Input: part model. Units: mm. Frame: model coordinates. Give positions to 0.01 mm unless a question says otherwise; leave off trailing zeros. Write each loop counter-clockwise with the first axis right and the second up, starting at its lowest first coordinate (ties: lowest second). Pieces come first, ordered by that corner, then holes. Notation, with made-up numbers: (59.25, 14.25) - (79.25, 14.25) arc R16 ccw to (79.25, 41.25) - close; hole circle Ø7 at (36, 88). An arc over 180 degrees is marked (long way). Answer as a JSON object with one key per item and string values. Group by question number.
from build123d import *

# Parameters (mm, degrees)
SKETCH2_R           = 1.5
SKETCH2_W           = 40
SKETCH2_H           = 20
SKETCH2_W_2         = 10
SKETCH2_H_2         = 3
BOSS_EXTRUDE1_DEPTH = 3


with BuildPart() as part:
    # Sketch2 → Boss-Extrude1 (new body)
    with BuildSketch(Plane(origin=(0, 0, 0), x_dir=(1, 0, 0), z_dir=(0, 1, 0))):
        Polygon((0, 15.5), (5, 15.5), (5, 47.5), (-45, 47.5), (-45, 15.5), (-40, 15.5), (-40, 0), (-36, 0), (-36, -3), (-26, -3), (-26, 0), (-21.5, 0), (-21.5, 3.1), (-22.8, 3.1), (-22.8, 5.6), (-21.5, 5.6), (-21.5, 9.4), (-18.5, 9.4), (-18.5, 5.6), (-17.2, 5.6), (-17.2, 3.1), (-18.5, 3.1), (-18.5, 0), (-14, 0), (-14, -3), (-4, -3), (-4, 0), (0, 0), align=None)
        with Locations(Location((-7.5, 15.5, 0), (0, 0, 270))):
            Circle(SKETCH2_R, mode=Mode.SUBTRACT)
        with Locations(Location((-32.5, 15.5, 0), (0, 0, 270))):
            Circle(SKETCH2_R, mode=Mode.SUBTRACT)
        with Locations(Location((-30.75, 7.9, 0), (0, 0, 270))):
            Circle(SKETCH2_R, mode=Mode.SUBTRACT)
        with Locations((-20, 31.5)):
            Rectangle(SKETCH2_W, SKETCH2_H, mode=Mode.SUBTRACT)
        with Locations((-20, 15.5)):
            Rectangle(SKETCH2_W_2, SKETCH2_H_2, mode=Mode.SUBTRACT)
        with Locations((-9, 7.9)):
            Rectangle(SKETCH2_W_2, SKETCH2_H_2, mode=Mode.SUBTRACT)
    extrude(amount=BOSS_EXTRUDE1_DEPTH)


solid = part.part
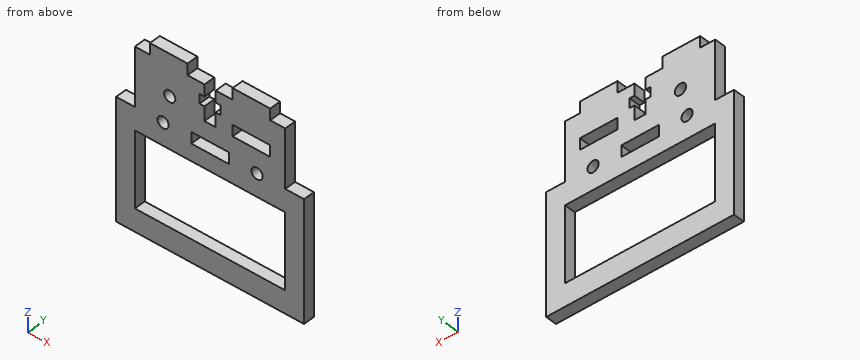
1) Cut plane D-D on y = 2.35. Count the separate pieces of the cut face and the enclosed holes in it, and give its area (3 significant figures).
2) Cut plane B-B on x = -7.5. Return the cut outline in (y, z), and give its area (3 significant figures).
3) Pin query (flat end, axial travel): P1, Ø1.5, axis at x = -24.5, y = 2, coming from the +Z side; P2, Ø0.7, axis at y = 2, z = -4, coming from the +X side; P3, Ø1.8, axis at x = -30.75, z = -7.9, coming from the +Y side. Return the tip coordinate at first contact, or that it passes through.
4) Cut plane A-A on z = -7.9. Return the cut outline in (x, y).
5) Line query: line 1 along X through (y, z) = (1.6, -7.9); line 2 along Z through (x, y) = (-10, 1.35); line 3 along Z through (x, y) = (-20, 2.45). Output: solid intervals per line, ascending. Write a range as from..to.
6) Cut plane C-C on z = -34.5. Return the cut outline in (x, y).
Filled in:
{
 "1": {"separate pieces": "1", "enclosed holes": "6", "area": "1,360 mm²"},
 "2": {"outline": "(0, -47.5) - (3, -47.5) - (3, -41.5) - (0, -41.5) - close; (0, -21.5) - (3, -21.5) - (3, -17) - (0, -17) - close; (0, -14) - (3, -14) - (3, -9.4) - (0, -9.4) - close; (0, -6.4) - (3, -6.4) - (3, 3) - (0, 3) - close", "area": "73.5 mm²"},
 "3": {"P1": "stops at z = 0", "P2": "stops at x = 0", "P3": "passes through"},
 "4": {"outline": "(-40, 0) - (-32.25, 0) - (-32.25, 3) - (-40, 3) - close; (-29.25, 0) - (-21.5, 0) - (-21.5, 3) - (-29.25, 3) - close; (-18.5, 0) - (-14, 0) - (-14, 3) - (-18.5, 3) - close; (-4, 0) - (0, 0) - (0, 3) - (-4, 3) - close"},
 "5": {"line 1": "x = -40..-32.25, -29.25..-21.5, -18.5..-14, -4..0", "line 2": "z = -47.5..-41.5, -21.5..-9.4, -6.4..3", "line 3": "z = -47.5..-41.5, -21.5..-17, -14..-9.4"},
 "6": {"outline": "(-45, 0) - (-40, 0) - (-40, 3) - (-45, 3) - close; (0, 0) - (5, 0) - (5, 3) - (0, 3) - close"}
}
